Part model, mm, in its own coordinate system. Face numbers are marked on the shaded views. Give positions to 0.01 mm unless a question says otherwise; leave off trailing zeros. Write each loop counter-clockwise with the first axis right and the second up, starting at its lowest first coordinate (ties: lowest second). Pieces come first, ordered by that corner, then holes. Notation, with made-up numbers: M -26.5,-26 L 21.5,-26 A28 cw 21.5,5 Z; hole C 67,-7.75 d9. An arc over 180 degrees is marked long. Use a Markdown table: item, result.
Autodesk Inventor part; units mm, degrees
ref_plane "YZ Plane" through (0, 0, 0) normal (1, 0, 0) x (0, 1, 0)
ref_plane "XZ Plane" through (0, 0, 0) normal (0, 1, 0) x (-1, 0, 0)
ref_plane "XY Plane" through (0, 0, 0) normal (0, 0, 1) x (1, 0, 0)
sketch "Sketch1" plane through (0, 0, 0) normal (0, 0, 1) x (1, 0, 0)
  line L0 (0, 0) -> (60, 0)
  line L1 (60, 0) -> (60, 47)
  line L2 (60, 47) -> (0, 47)
  line L3 (0, 47) -> (0, 0)
  circle A0 centre (30, 23.5) radius 18.5
  line L4 (11.5, 42) -> (48.5, 42) construction
  line L5 (48.5, 42) -> (48.5, 5) construction
  line L6 (48.5, 5) -> (11.5, 5) construction
  line L7 (11.5, 5) -> (11.5, 42) construction
  point P0 (60, 23.5)
  point P1 (30, 47)
  dimension "d0" = 37
  dimension "d1" = 5
  dimension "d5" = 60
extrude "Extrusion1" add sketch "Sketch1" along normal blind 22.5
fillet "Fillet1" radius 4 4 edges at (60, 47, 11.25) (60, 0, 11.25) (0, 0, 11.25) (0, 47, 11.25)
properties part number "Gearbox Mount"
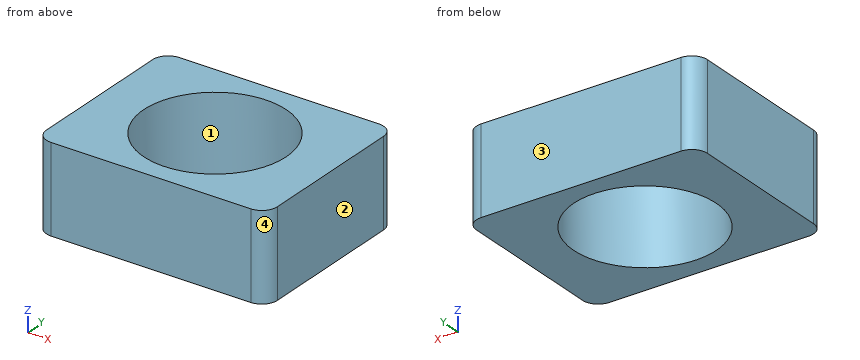
1. Drill centre lines: L1, parallel to Y at x = 30, z = 6.25; L2, parallel to X at y = 23, z = 14.75; L3, parallel to X at y = 29.5, z = 18.25. Where is each one in solid material? Low to high.
Findings below:
| item | result |
|---|---|
| L1 | 0 to 5, 42 to 47 |
| L2 | 0 to 11.51, 48.49 to 60 |
| L3 | 0 to 12.5, 47.5 to 60 |
2. Two-plate mould, pull along Y, no slides. Class the marked faces 1, 2, 3 and 4: released by +Y, released by -Y, zero draft, split by the parting line, or undercut.
Findings below:
| item | result |
|---|---|
| face 1 | undercut |
| face 2 | zero draft |
| face 3 | released by +Y |
| face 4 | released by -Y |
3. Cut at C-C, the plane y = 23.5. Give the cut face in (x, z).
Findings below:
| item | result |
|---|---|
| outline | M 0,0 L 11.5,0 L 11.5,22.5 L 0,22.5 Z; M 48.5,0 L 60,0 L 60,22.5 L 48.5,22.5 Z |
4. Cut at B-B, the plane z = 5.75. Give the cut face in (x, y).
Findings below:
| item | result |
|---|---|
| outline | M 0,4 A4 ccw 4,0 L 56,0 A4 ccw 60,4 L 60,43 A4 ccw 56,47 L 4,47 A4 ccw 0,43 Z; hole C 30,23.5 d37 |
5. Cut at A-A, the plane x = 30. Give the cut face in (y, z).
Findings below:
| item | result |
|---|---|
| outline | M 0,0 L 5,0 L 5,22.5 L 0,22.5 Z; M 42,0 L 47,0 L 47,22.5 L 42,22.5 Z |
